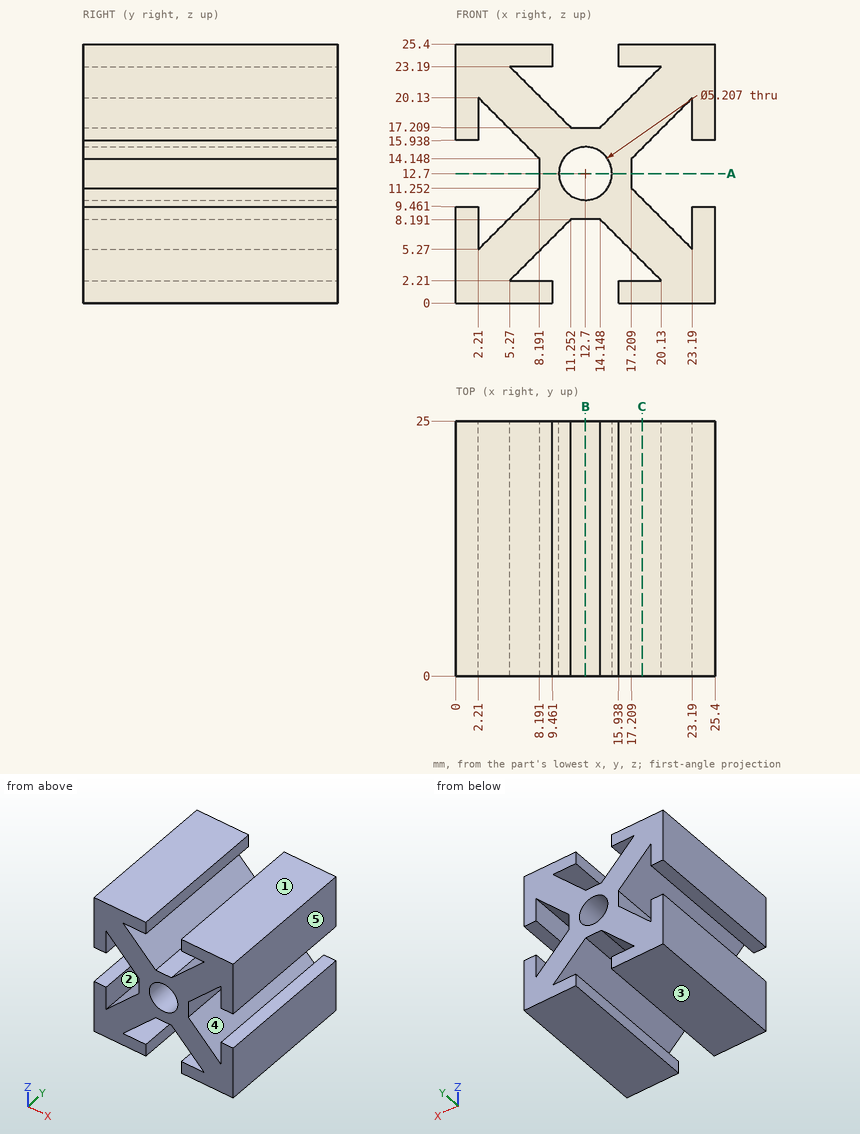
Can you work these out from the drawing? Everything is in mm from the part's minimum corner. A direction names the side the tool comes from. Give positions to 0.01 mm unless a question says otherwise; leave off trailing zeros. Order: outer loops, then holes, each group sorted by start corner. A loop starts at its lowest first (then second) coordinate and runs counter-clockwise, first axis right, second up. Notation, with made-up numbers: M 74.25,82 L 82.25,82 A15 ccw 82.25,91 Z; hole C -29,5 d1. An arc over 180 degrees is marked long. Use a Markdown table: item, result. Add a question column.
Item 1: Will these pins go through, and if not, where does the flat tip stop? pin 1 (3 mm diameter, centred on x = 12, y = 14, fed in from -Z); pin 2 (2 mm diameter, centred on y = 13.5, z = 7, fed in from -X); pin 3 (2.5 mm diameter, centred on y = 8, z = 13, fed in from -X); pin 4 (3 mm diameter, centred on y = 16, z = 13, fed in from +X).
Item 2: We'd pull the mould along X, two halves only. Please class the marked faces 3, 4 and 5: +X half, -X half, draft (parallel to the pull), parting line (faces both ways), or undercut.
Item 3: If I drill on L1, parallel to Z at x = 12.7, y = 15; L2, parallel to X at y = 17.5, z = 2; L3, parallel to X at y = 19, z = 7, over which ranges is the centre line in solid material (lowest first)? Write a range as [from, to].
Item 4: Suppose I cut it at A-A (z = 12.7). List the corners of the cut face in (x, y) for me.
Item 5: For the marked faces 1 and 2, which set-ups out of +Z, -Z, +X, -X, +Y, -Y let a thin tool reach every point of the face, with its end or its side?
Item 6: Suppose I cut it at C-C (x = 18.25). List the corners of the cut face in (y, z) for me.
Item 7: Suppose I cut it at B-B (x = 12.7). List the corners of the cut face in (y, z) for me.
Answer sheet:
| question | item | result |
|---|---|---|
| 1 | pin 1 | stops at z = 7.44 |
| 1 | pin 2 | stops at x = 0 |
| 1 | pin 3 | stops at x = 8.09 |
| 1 | pin 4 | stops at x = 17.56 |
| 2 | face 3 | draft |
| 2 | face 4 | undercut |
| 2 | face 5 | +X half |
| 3 | L1 | z = [8.19, 10.1], [15.3, 17.21] |
| 3 | L2 | x = [0, 9.46], [15.94, 25.4] |
| 3 | L3 | x = [0, 2.21], [3.94, 10.06], [15.34, 21.46], [23.19, 25.4] |
| 4 | outline | M 8.19,0 L 10.1,0 L 10.1,25 L 8.19,25 Z; M 15.3,0 L 17.21,0 L 17.21,25 L 15.3,25 Z |
| 5 | face 1 | +Z, +X, -X, +Y, -Y |
| 5 | face 2 | +Y, -Y |
| 6 | outline | M 0,0 L 25,0 L 25,2.21 L 0,2.21 Z; M 0,4.09 L 25,4.09 L 25,10.21 L 0,10.21 Z; M 0,15.19 L 25,15.19 L 25,21.31 L 0,21.31 Z; M 0,23.19 L 25,23.19 L 25,25.4 L 0,25.4 Z |
| 7 | outline | M 0,8.19 L 25,8.19 L 25,10.1 L 0,10.1 Z; M 0,15.3 L 25,15.3 L 25,17.21 L 0,17.21 Z |
